Autodesk Inventor part; units mm, degrees
ref_plane "YZ Plane" through (0, 0, 0) normal (1, 0, 0) x (0, 1, 0)
ref_plane "XZ Plane" through (0, 0, 0) normal (0, 1, 0) x (-1, 0, 0)
ref_plane "XY Plane" through (0, 0, 0) normal (0, 0, 1) x (1, 0, 0)
sketch "スケッチ1" plane through (0, 0, 0) normal (0, 0, 1) x (1, 0, 0)
  line L0 (99, -354) -> (-99, -354)
  line L1 (-99, -354) -> (-99, 354)
  line L2 (-99, 354) -> (99, 354)
  line L3 (99, 354) -> (99, -354)
  line L4 (99, -354) -> (-99, 354) construction
  line L5 (-99, -354) -> (99, 354) construction
  point P0 (0, 0)
  dimension "d0" = 198
  dimension "d1" = 708
extrude "押し出し1" add sketch "スケッチ1" along normal blind 3
sketch "スケッチ4" plane through (0, 0, 0) normal (0, 0, -1) x (-1, 0, 0)
  line L0 (99, -354) -> (-99, -354)
  line L1 (99, 354) -> (99, -354)
  line L2 (-99, 354) -> (99, 354)
  line L3 (-99, -354) -> (-99, 354)
  line L4 (-88, 343) -> (88, 343)
  line L5 (88, 343) -> (88, -343)
  line L6 (88, -343) -> (-88, -343)
  line L7 (-88, -343) -> (-88, 343)
  line L8 (-88, -256.5) -> (88, -256.5)
  line L9 (88, -256.5) -> (88, 256.5)
  line L10 (88, 256.5) -> (-88, 256.5)
  line L11 (-88, 256.5) -> (-88, -256.5)
  point P0 (0, 0)
  point P1 (0, -343)
  point P2 (0, 343)
  point P3 (-88, 0)
  point P4 (88, 0)
  dimension "d32" = 11
  dimension "d33" = 86.5
  dimension "d34" = 86.5
hole "穴3" at (0, -343, 0) at (0, 343, 0) at (88, 0, 0) at (-88, 0, 0) at (-88, -256.5, 0) at (88, -256.5, 0) at (88, 256.5, 0) at (-88, 256.5, 0) direction (0, 0, 1) diameter 6 end through all
sketch "スケッチ5" plane through (0, 0, 3) normal (0, 0, 1) x (1, 0, 0)
  circle A0 centre (88, 256.5) radius 3
  circle A1 centre (-88, -256.5) radius 3
  circle A2 centre (88, 0) radius 3
  circle A3 centre (0, -343) radius 3
  circle A4 centre (0, 343) radius 3
  circle A5 centre (-88, 0) radius 3
  circle A6 centre (88, -256.5) radius 3
  circle A7 centre (-88, 256.5) radius 3
  line L0 (-99, -354) -> (99, -354)
  line L1 (99, -354) -> (99, 354)
  line L2 (99, 354) -> (-99, 354)
  line L3 (-99, 354) -> (-99, -354)
  line L4 (-25, -45) -> (25, -45)
  line L5 (25, -45) -> (25, -195)
  line L6 (25, -195) -> (-25, -195)
  line L7 (-25, -195) -> (-25, -45)
  line L8 (-25, -45) -> (25, -195) construction
  line L9 (25, -45) -> (-25, -195) construction
  point P0 (0, 0)
  point P1 (0, -120)
  point P2 (0, -120)
  dimension "d42" = 150
  dimension "d43" = 50
  dimension "d44" = 120
hole "穴4" at (-25, -45, 3) at (25, -45, 3) at (-25, -195, 3) at (25, -195, 3) direction (0, 0, -1) diameter 4.2 end through all
sketch "スケッチ6" plane through (0, 0, 3) normal (0, 0, 1) x (1, 0, 0)
  circle A0 centre (-25, -195) radius 2.1
  circle A1 centre (-25, -45) radius 2.1
  circle A2 centre (25, -45) radius 2.1
  circle A3 centre (25, -195) radius 2.1
  circle A4 centre (88, 256.5) radius 3
  circle A5 centre (-88, -256.5) radius 3
  circle A6 centre (88, 0) radius 3
  circle A7 centre (0, -343) radius 3
  circle A8 centre (0, 343) radius 3
  circle A9 centre (-88, 0) radius 3
  circle A10 centre (88, -256.5) radius 3
  circle A11 centre (-88, 256.5) radius 3
  line L0 (-99, -354) -> (99, -354)
  line L1 (99, -354) -> (99, 354)
  line L2 (99, 354) -> (-99, 354)
  line L3 (-99, 354) -> (-99, -354)
  line L4 (11, 316.5) -> (39, 316.5)
  line L5 (39, 316.5) -> (39, 269.5)
  line L6 (39, 269.5) -> (11, 269.5)
  line L7 (11, 269.5) -> (11, 316.5)
  line L8 (11, 316.5) -> (39, 269.5) construction
  line L9 (39, 316.5) -> (11, 269.5) construction
  line L10 (-39, 316.5) -> (-11, 316.5)
  line L11 (-11, 316.5) -> (-11, 269.5)
  line L12 (-11, 269.5) -> (-39, 269.5)
  line L13 (-39, 269.5) -> (-39, 316.5)
  line L14 (-39, 316.5) -> (-11, 269.5) construction
  line L15 (-11, 316.5) -> (-39, 269.5) construction
  line L16 (25, 321) -> (-25, 321)
  line L17 (-25, 321) -> (-25, 265)
  line L18 (-25, 265) -> (25, 265)
  line L19 (25, 265) -> (25, 321)
  circle A12 centre (25, 321) radius 1.6
  circle A13 centre (25, 265) radius 1.6
  circle A14 centre (-25, 265) radius 1.6
  circle A15 centre (-25, 321) radius 1.6
  point P0 (0, 0)
  point P1 (25, 293)
  point P2 (-25, 293)
  point P3 (-25, 293)
  point P4 (25, 293)
  point P5 (-25, 293)
  point P6 (25, 293)
  point P7 (-23.4, 265)
  point P8 (-25, 266.6)
  dimension "d52" = 47
  dimension "d53" = 28
  dimension "d54" = 28
  dimension "d55" = 50
  dimension "d56" = 25
  dimension "d57" = 50
  dimension "d58" = 56
  dimension "d59" = 28
  dimension "d60" = 3.2
  dimension "d61" = 3.2
  dimension "d62" = 3.2
  dimension "d63" = 3.2
extrude "押し出し2" cut sketch "スケッチ6" against normal blind 10 contours L4 L19 L6 L7 | L4 L5 L6 L19 | A12 L16 L19 | L19 L16 A12 | A13 L18 L19 | L19 L18 A13 | A15 L17 L16 | L16 L17 A15 | A14 L17 L18 | L18 L17 A14 | L17 L12 L13 L10 | L10 L11 L12 L17
sketch "スケッチ7" plane through (0, 0, 3) normal (0, 0, 1) x (1, 0, 0)
  circle A0 centre (0, 214) radius 11.15
  line L0 (99, 354) -> (-99, 354)
  point P0 (0, 0)
  dimension "d66" = 22.3
  dimension "d67" = 140
extrude "押し出し3" cut sketch "スケッチ7" against normal blind 10
sketch "スケッチ8" plane through (0, 0, 3) normal (0, 0, 1) x (1, 0, 0)
  line L0 (4.8167, 215.6) -> (13.35, 215.6)
  line L1 (13.35, 215.6) -> (13.35, 212.4)
  line L2 (13.35, 212.4) -> (4.8167, 212.4)
  line L3 (4.8167, 212.4) -> (4.8167, 215.6)
  circle A0 centre (0, 214) radius 11.15
  circle A1 centre (0, 214) radius 11.15
  point P0 (0, 0)
  point P1 (-11.15, 214)
  point P2 (11.0346, 215.6)
  point P3 (11.0346, 212.4)
  dimension "d70" = 3.2
  dimension "d71" = 1.6
  dimension "d72" = 24.5
extrude "押し出し4" cut sketch "スケッチ8" against normal blind 10 contours L0 L1 L2 A0
sketch "スケッチ9" plane through (0, 0, 3) normal (0, 0, 1) x (1, 0, 0)
  point P0 (0, 0)
  point P1 (70, 100)
  point P2 (-70, 100)
  point P3 (0, 100)
  dimension "d75" = 140
  dimension "d76" = 70
  dimension "d77" = 100
hole "穴5" at (70, 100, 3) at (-70, 100, 3) at (0, 100, 3) direction (0, 0, -1) diameter 4.2 end through all
sketch "スケッチ10" plane through (0, 0, 3) normal (0, 0, 1) x (1, 0, 0)
  circle A0 centre (-70, 100) radius 2.1
  circle A1 centre (70, 100) radius 2.1
  circle A2 centre (0, 100) radius 2.1
  line L0 (13.35, 212.4) -> (11.0346, 212.4)
  arc A3 (11.0346, 215.6) -> (11.0346, 212.4) centre (0, 214) ccw
  line L1 (11.0346, 215.6) -> (13.35, 215.6)
  line L2 (13.35, 215.6) -> (13.35, 212.4)
  circle A4 centre (25, 265) radius 1.6
  line L3 (11, 269.5) -> (11, 316.5)
  line L4 (11, 316.5) -> (39, 316.5)
  line L5 (39, 316.5) -> (39, 269.5)
  line L6 (39, 269.5) -> (11, 269.5)
  circle A5 centre (-25, 321) radius 1.6
  circle A6 centre (-25, 265) radius 1.6
  circle A7 centre (25, 321) radius 1.6
  line L7 (-11, 269.5) -> (-39, 269.5)
  line L8 (-39, 269.5) -> (-39, 316.5)
  line L9 (-39, 316.5) -> (-11, 316.5)
  line L10 (-11, 316.5) -> (-11, 269.5)
  circle A8 centre (-25, -195) radius 2.1
  circle A9 centre (-25, -45) radius 2.1
  circle A10 centre (25, -45) radius 2.1
  circle A11 centre (25, -195) radius 2.1
  circle A12 centre (88, 256.5) radius 3
  circle A13 centre (-88, -256.5) radius 3
  circle A14 centre (88, 0) radius 3
  circle A15 centre (0, -343) radius 3
  circle A16 centre (0, 343) radius 3
  circle A17 centre (-88, 0) radius 3
  circle A18 centre (88, -256.5) radius 3
  circle A19 centre (-88, 256.5) radius 3
  line L11 (-99, -354) -> (99, -354)
  line L12 (99, -354) -> (99, 354)
  line L13 (99, 354) -> (-99, 354)
  line L14 (-99, 354) -> (-99, -354)
  point P0 (0, 0)
properties part number "Cut_A"
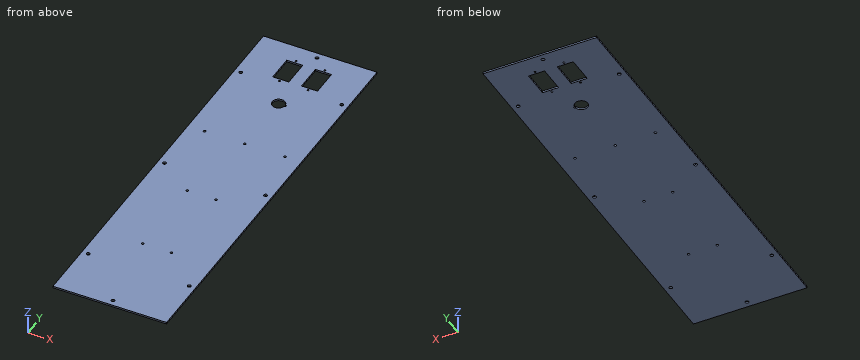
Check sheet for the modelled part. Datum: model origin and axes. Units: mm. Give positions to 0.01 mm unless a question says otherwise; leave off trailing zeros. Answer in a Markdown table with one row per item.
1) Cross-section at A-A (z = 0.95). Count the separate pieces of the cut face and the enclosed holes in it, plus the area to 3 significant figures.
Solutions:
| item | result |
|---|---|
| separate pieces | 1 |
| enclosed holes | 22 |
| area | 137,000 mm^2 |
2) Thickness scan on line 1 (X direction, y = 0, z = 2.25); line 2 (Y direction, x = 0, z = 1.45); line 3 (Y direction, x = -25, z = 2). Record the ranges inside material, lowest first.
Solutions:
| item | result |
|---|---|
| line 1 | x = -99 to -91, -85 to 85, 91 to 99 |
| line 2 | y = -354 to -346, -340 to 97.9, 102.1 to 202.85, 225.15 to 340, 346 to 354 |
| line 3 | y = -354 to -197.1, -192.9 to -47.1, -42.9 to 263.4, 266.6 to 269.5, 316.5 to 319.4, 322.6 to 354 |
3) Depth check by flat-ended pin: pin 1 (2.5 mm diameter, centred on x = 25, y = -45, fed in from -Z); pin 2 (8 mm diameter, centred on x = -88, y = 0, fed in from +Z). Enter the tip coordinate at first touch or a pass-through.
Solutions:
| item | result |
|---|---|
| pin 1 | passes through |
| pin 2 | stops at z = 3 |
